```python
from build123d import *

# Parameters (mm, degrees)
SKETCH1_W            = 80
SKETCH1_H            = 10
BOSS_EXTRUDE1_DEPTH  = 5
SKETCH2_W            = 74
SKETCH2_H            = 4.3
CUT_EXTRUDE1_DEPTH   = 5
FILLET1_R            = 4
FILLET2_R            = 2
SKETCH3_W            = 5
SKETCH3_H            = 5
BOSS_EXTRUDE2_DEPTH  = 50
FILLET1_OF_MIRROR1_R = 4
FILLET2_OF_MIRROR1_R = 2


with BuildPart() as part:
    # Sketch1 → Boss-Extrude1 (new body)
    with BuildSketch(Plane(origin=(0, 0, 0), x_dir=(1, 0, 0), z_dir=(0, 1, 0))):
        Rectangle(SKETCH1_W, SKETCH1_H)
    boss_extrude1 = extrude(amount=BOSS_EXTRUDE1_DEPTH)

    # Sketch2 → Cut-Extrude1 (cut)
    with BuildSketch(Plane(origin=(0, 5, 0), x_dir=(1, 0, 0), z_dir=(0, 1, 0))):
        Rectangle(SKETCH2_W, SKETCH2_H)
    cut_extrude1 = extrude(amount=-CUT_EXTRUDE1_DEPTH, mode=Mode.SUBTRACT)

    # Fillet1
    fillet1_edges = [part.edges().sort_by_distance(p)[0] for p in [
        (40, 2.5, 5),
        (-40, 2.5, 5),
        (-40, 2.5, -5),
        (40, 2.5, -5),
    ]]
    fillet(fillet1_edges, radius=FILLET1_R)

    # Fillet2
    fillet2_edges = [part.edges().sort_by_distance(p)[0] for p in [
        (37, 2.5, -2.15),
        (37, 2.5, 2.15),
        (-37, 2.5, 2.15),
        (-37, 2.5, -2.15),
    ]]
    fillet(fillet2_edges, radius=FILLET2_R)

    # Sketch3 → Boss-Extrude2 (add)
    with BuildSketch(Plane(origin=(0, 0, -5), x_dir=(-1, 0, 0), z_dir=(0, 0, -1))):
        with Locations((-33.5, 2.5)):
            Rectangle(SKETCH3_W, SKETCH3_H)
        with Locations((33.5, 2.5)):
            Rectangle(SKETCH3_W, SKETCH3_H)
    extrude(amount=BOSS_EXTRUDE2_DEPTH)


with BuildPart() as mirror1_1:
    # Mirror1: Boss-Extrude1 across plane
    add(boss_extrude1.mirror(Plane(origin=(0, 0, -30), x_dir=(1, 0, 0), z_dir=(0, 0, -1))))

    # Mirror1 2: Cut-Extrude1 across plane
    add(cut_extrude1.mirror(Plane(origin=(0, 0, -30), x_dir=(1, 0, 0), z_dir=(0, 0, -1))), mode=Mode.SUBTRACT)

    # Fillet1 of Mirror1
    fillet1_of_mirror1_edges = [mirror1_1.edges().sort_by_distance(p)[0] for p in [
        (40, 2.5, -65),
        (-40, 2.5, -65),
        (-40, 2.5, -55),
        (40, 2.5, -55),
    ]]
    fillet(fillet1_of_mirror1_edges, radius=FILLET1_OF_MIRROR1_R)

    # Fillet2 of Mirror1
    fillet2_of_mirror1_edges = [mirror1_1.edges().sort_by_distance(p)[0] for p in [
        (37, 2.5, -57.85),
        (37, 2.5, -62.15),
        (-37, 2.5, -62.15),
        (-37, 2.5, -57.85),
    ]]
    fillet(fillet2_of_mirror1_edges, radius=FILLET2_OF_MIRROR1_R)


with BuildPart() as part_1:
    add(part.part)

    # Mirror1 united with what the copies touc: union Mirror1_1
    add(mirror1_1.part)


solid = part_1.part
```
The model under review builds one solid part; all positions refer to its coordinate system, in mm. A direction names the side the tool comes from. Coordinates: 2 decimals unless noted, no trailing zeros. Write each loop counter-clockwise with the first axis right and the second up, starting at its lowest first coordinate (ties: lowest second). Pieces come first, ordered by that corner, then holes. Notation, with made-up numbers: (49.5, -6.75) -> (108.5, -6.75) arc R28 ccw to (108.5, 13.25) -> close; hole circle Ø2 at (-4.75, 81). An arc over 180 degrees is marked (long way). One line per item, written item: value. Start each with the question number.
Q1. The part is to be moulded in two halves that separate along Z. For faces 4 (the face through (0, 2, -5)), 5 (the face through (38.797, 2.535, -63.859)), 6 (the face through (3, 0, -56)), 7 (the face through (38.797, 2.535, 3.859)), say which applies: +Z half, -Z half, draft (parallel to the pull), parting line (faces both ways), or undercut.
Q2. Add section C-C, the plane y = 4.25. Count the separate pieces of the cut face and the enclosed holes in it, then the cut area to 3 significant figures.
Q3. Add section B-B, the plane z = -36.5. Give the boundary of the cut face in (x, y), then the cut area to 3 significant figures.
Q4. For faces 1 (the face through (-38.859, 2.535, -56.203)), 2 (the face through (36.4, 2.46, -61.58)), 3 (the face through (38.797, 2.535, -56.141)), list the 3-axis set-ups (+Z, -Z, +X, -X, +Y, -Y) from which the entire face can be reached by the end or side of a thin tool; tool diameter is ignored.
Q5. Add section A-A, the plane x = -26. Give the boundary of the cut face in (y, z), then the cut area to 3 significant figures.
Q6. To check wall thickness, follow probe 1 along Z at (x, y) = (22.5, 4.2); probe 2 along X at (y, z) = (1.05, -35); probe 3 along X at (y, z) = (3, 0). State the ranges of each line that lie inside material, in increasing order.
Response:
1. face 4: undercut
1. face 5: -Z half
1. face 6: draft
1. face 7: +Z half
2. separate pieces: 1
2. enclosed holes: 3
2. area: 1,440 mm²
3. outline: (-36, 0) -> (-31, 0) -> (-31, 5) -> (-36, 5) -> close; (31, 0) -> (36, 0) -> (36, 5) -> (31, 5) -> close
3. area: 50.0 mm²
4. face 1: -X, +Y, -Y
4. face 2: +Y, -Y
4. face 3: +X, +Y, -Y
5. outline: (0, -65) -> (5, -65) -> (5, -62.15) -> (0, -62.15) -> close; (0, -57.85) -> (5, -57.85) -> (5, -55) -> (0, -55) -> close; (0, -5) -> (5, -5) -> (5, -2.15) -> (0, -2.15) -> close; (0, 2.15) -> (5, 2.15) -> (5, 5) -> (0, 5) -> close
5. area: 57.0 mm²
6. probe 1: -65 to -62.15, -57.85 to -55, -5 to -2.15, 2.15 to 5
6. probe 2: -36 to -31, 31 to 36
6. probe 3: -40 to -37, 37 to 40
